```python
from build123d import *

# Parameters (mm, degrees)
F3_W     = 10.5
F3_H     = 15.8350876221
F3_R     = 2.7
F4_DEPTH = 3
F5_R     = 1
F7_DEPTH = 3
F8_R     = 1
F9_SIZE  = 1


with BuildPart() as f2:
    # F0 (on Front) → F2 (revolve)
    with BuildSketch(Plane.XZ):
        Polygon((4.3, 7), (4.3, 0), (10, 0), (10, 11), (9.5, 17.5), (2.7, 17.5), (2.7, 11.5), align=None)
    revolve(axis=Axis((0, 0, 12.8003526479), (0, 0, -1)))

    # F3 (on face) → F4 (join)
    with BuildSketch(Plane.XY.offset(17.5)):
        Rectangle(F3_W, F3_H)
        Circle(F3_R, mode=Mode.SUBTRACT)
    extrude(amount=F4_DEPTH)

    # F5
    f5_edges = [f2.edges().sort_by_distance(p)[0] for p in [
        (-5.25, -7.917544, 19),
        (5.25, -7.917544, 19),
    ]]
    fillet(f5_edges, radius=F5_R)

    # F6 (on face) → F7 (join)
    with BuildSketch(Plane.XY.offset(17.5)):
        with BuildLine():
            Line((-5.25, 7.9175438111), (5.25, 7.9175438111))
            ThreePointArc((5.25, 7.9175438111), (0, 9.5), (-5.25, 7.9175438111))
        make_face()
    extrude(amount=F7_DEPTH)

    # F8
    f8_edges = [f2.edges().sort_by_distance(p)[0] for p in [
        (5.25, 7.917544, 19),
        (-5.25, 7.917544, 19),
    ]]
    fillet(f8_edges, radius=F8_R)

    # F9
    f9_edges = [f2.edges().sort_by_distance(p)[0] for p in [
        (-2.7, 0, 20.5),
        (2.7, 0, 19),
    ]]
    chamfer(f9_edges, length=F9_SIZE)


solid = f2.part
```
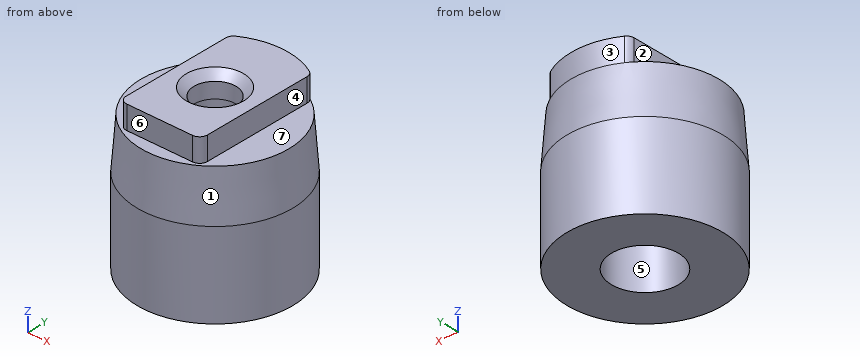
Geometry check sheet. Reference: the model listing, model coordinates, mm. Face numbers are marked on the shaded views. A direction names the side the tool comes from. Coordinates: 2 decimals unless noted, no trailing zeros. Order: outer loops, then holes, each group sorted by start corner. A loop starts at its lowest first (then second) coordinate and runs counter-clockwise, first axis right, second up.
Item 1: Section check D-D (z = 13.25). Enter the section's corners in (x, y), plus the area to 3 significant figures.
Item 2: Depth check by flat-ended pin: pin 1 (6 mm diameter, centred on x = 0, y = 0, fed in from +Z); pin 2 (4 mm diameter, centred on x = 1, z = 16.5, fed in from +Y); pin 3 (7 mm diameter, centred on x = 0, y = 0, fed in from +Z). Enter the tip coordinate at first touch or a pass-through.
Item 3: Section check C-C (z = 5). Enter the section's corners in (x, y).
Item 4: Tool access check on the marked faces 1, 2, 3 and 4. Record the directions out of +Z, -Z, +X, -X, +Y, -Y that give a thin tool (end or side, any length) a straight path to the whole face; none if there is none.
Item 5: Scan lines: line 1 along X through (y, z) = (0, 18.2); line 2 along Y through (x, z) = (0, 18.5); line 3 along X through (y, z) = (0, 3.5). Record each from-to range of solid material in increasing order.
Item 6: Section check B-B (y = 0). Enter the section's corners in (x, z).
Item 7: Mould release check, pull along Y, two halves, no side actions. Record for the marked faces 5, 6 and 7: released by +Y, released by -Y, zero draft, split by the parting line, or undercut.
Item 8: Section check A-A (x = 0). Enter the section's corners in (y, z).
Check sheet entries:
1. outline: circle Ø19.65 at (0, 0); hole circle Ø5.4 at (0, 0)
1. area: 280 mm2
2. pin 1: stops at z = 19.8
2. pin 2: stops at y = 9.72
2. pin 3: stops at z = 20.3
3. outline: circle Ø20 at (0, 0); hole circle Ø8.6 at (0, 0)
4. face 1: +Z
4. face 2: +Z, -X, +Y, -Y
4. face 3: +Z, +Y
4. face 4: +Z, +X, +Y, -Y
5. line 1: x = -5.25 to -2.7, 2.7 to 5.25
5. line 2: y = -7.92 to -2.7, 2.7 to 9.5
5. line 3: x = -10 to -4.3, 4.3 to 10
6. outline: (-10, 0) - (-4.3, 0) - (-4.3, 7) - (-2.7, 11.5) - (-2.7, 19.5) - (-3.7, 20.5) - (-5.25, 20.5) - (-5.25, 17.5) - (-9.5, 17.5) - (-10, 11) - close; (2.7, 11.5) - (4.3, 7) - (4.3, 0) - (10, 0) - (10, 11) - (9.5, 17.5) - (5.25, 17.5) - (5.25, 20.5) - (3.7, 20.5) - (2.7, 19.5) - close
7. face 5: undercut
7. face 6: released by -Y
7. face 7: zero draft
8. outline: (-10, 0) - (-4.3, 0) - (-4.3, 7) - (-2.7, 11.5) - (-2.7, 19.5) - (-3.7, 20.5) - (-7.92, 20.5) - (-7.92, 17.5) - (-9.5, 17.5) - (-10, 11) - close; (2.7, 11.5) - (4.3, 7) - (4.3, 0) - (10, 0) - (10, 11) - (9.5, 17.5) - (9.5, 20.5) - (3.7, 20.5) - (2.7, 19.5) - close
